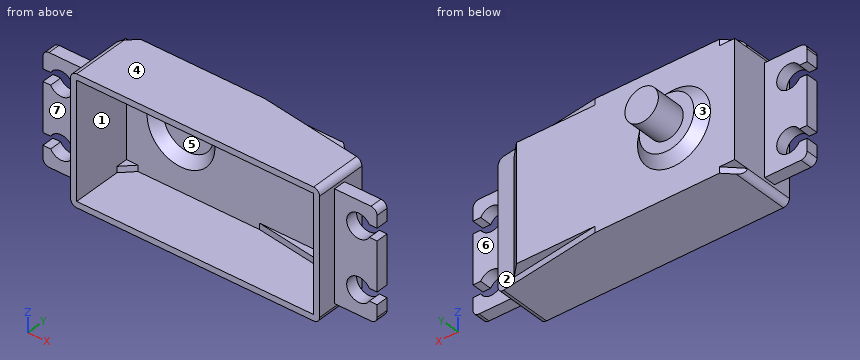
from build123d import *

# Parameters (mm, degrees)
BOSS_EXTRU_1_DEPTH      = 11
ENL_V_MAT_EXTRU_1_DEPTH = 48.360320945
ESQUISSE6_W             = 24.300768243
ESQUISSE6_H             = 19
BOSS_EXTRU_2_DEPTH      = 5
CHANFREIN1_SIZE         = 2.08
ESQUISSE7_R             = 6
BOSS_EXTRU_3_DEPTH      = 1.5
CHANFREIN2_SIZE         = 1.5
ENL_V_MAT_EXTRU_2_DEPTH = 1
ENL_V_MAT_EXTRU_3_DEPTH = 1
ESQUISSE11_W            = 18
ESQUISSE11_H            = 2
BOSS_EXTRU_4_DEPTH      = 7
ENL_V_MAT_EXTRU_5_DEPTH = 47.671725916
CONG_1_R                = 1
CONG_1_OF_SYM_TRIE1_R   = 1
COQUE1_START            = -20
COQUE1_DEPTH            = 19
COQUE1_START_2          = -19
COQUE1_2_DEPTH          = 17
ESQUISSE18_R            = 2.75
BOSS_EXTRU_5_DEPTH      = 5


with BuildPart() as part:
    # Esquisse3 → Boss.-Extru.1 (new body)
    with BuildSketch(Plane(origin=(0, 0, 0), x_dir=(1, 0, 0), z_dir=(0, 1, 0))):
        with BuildLine():
            Line((1, 0), (40, 0))
            ThreePointArc((40, 0), (40.707106781, 0.292893219), (41, 1))
            Line((41, 1), (41, 20))
            ThreePointArc((41, 20), (40.707106781, 20.707106781), (40, 21))
            Line((40, 21), (1, 21))
            ThreePointArc((1, 21), (0.292893219, 20.707106781), (0, 20))
            Line((0, 20), (0, 1))
            ThreePointArc((0, 1), (0.292893219, 0.292893219), (1, 0))
        make_face()
    extrude(amount=BOSS_EXTRU_1_DEPTH)

    # Esquisse4 → Enlèv. mat.-Extru.1 (cut, through all)
    with BuildSketch(Plane.XY):
        Polygon((41, 11), (23, 11), (41, 8.5), align=None)
    extrude(amount=-ENL_V_MAT_EXTRU_1_DEPTH, mode=Mode.SUBTRACT)

    # Esquisse6 → Boss.-Extru.2 (add)
    with BuildSketch(Plane(origin=(0, 11, 0), x_dir=(1, 0, 0), z_dir=(0, 1, 0))):
        with Locations((25.849615878, 10.5)):
            Rectangle(ESQUISSE6_W, ESQUISSE6_H)
    extrude(amount=-BOSS_EXTRU_2_DEPTH)

    # Chanfrein1
    chanfrein1_edges = [part.edges().sort_by_distance(p)[0] for p in [
        (38, 11, -10.5),
    ]]
    chamfer(chanfrein1_edges, length=CHANFREIN1_SIZE)

    # Esquisse7 → Boss.-Extru.3 (add)
    with BuildSketch(Plane(origin=(0, 11, 0), x_dir=(1, 0, 0), z_dir=(0, 1, 0))):
        with Locations(Location((10, 10.5, 0), (0, 0, 90))):
            Circle(ESQUISSE7_R)
    extrude(amount=BOSS_EXTRU_3_DEPTH)

    # Chanfrein2
    chanfrein2_edges = [part.edges().sort_by_distance(p)[0] for p in [
        (10, 12.5, -4.5),
    ]]
    chamfer(chanfrein2_edges, length=CHANFREIN2_SIZE - 0.0001)  # a hair under: the kernel refuses the full size

    # Esquisse8 → Enlèv. mat.-Extru.2 (cut)
    with BuildSketch(Plane.XY):
        Polygon((0, 11), (2.5, 11), (0, 8.5), align=None)
    extrude(amount=-ENL_V_MAT_EXTRU_2_DEPTH, mode=Mode.SUBTRACT)

    # Esquisse9 → Enlèv. mat.-Extru.3 (cut)
    with BuildSketch(Plane(origin=(0, 0, -21), x_dir=(-1, 0, 0), z_dir=(0, 0, -1))):
        Polygon((0, 11), (-2.5, 11), (0, 8.5), align=None)
    extrude(amount=-ENL_V_MAT_EXTRU_3_DEPTH, mode=Mode.SUBTRACT)

    # Esquisse11 → Boss.-Extru.4 (add)
    with BuildSketch(Plane.ZY):
        with Locations((-10.5, 4)):
            Rectangle(ESQUISSE11_W, ESQUISSE11_H)
    boss_extru_4 = extrude(amount=BOSS_EXTRU_4_DEPTH)

    # Esquisse15 → Enlèv. mat.-Extru.5 (cut, through all)
    with BuildSketch(Plane(origin=(0, 5, 0), x_dir=(1, 0, 0), z_dir=(0, 1, 0))):
        with BuildLine():
            Line((-9.636099445, 16.5), (-5.732050808, 16.5))
            ThreePointArc((-5.732050808, 16.5), (-2, 15.5), (-5.732050808, 14.5))
            Line((-5.732050808, 14.5), (-9.636099445, 14.5))
            Line((-9.636099445, 14.5), (-9.636099445, 16.5))
        make_face()
        with BuildLine():
            Line((-9.636099445, 4.5), (-5.732050808, 4.5))
            ThreePointArc((-5.732050808, 4.5), (-2, 5.5), (-5.732050808, 6.5))
            Line((-5.732050808, 6.5), (-9.636099445, 6.5))
            Line((-9.636099445, 6.5), (-9.636099445, 4.5))
        make_face()
    enl_v_mat_extru_5 = extrude(amount=-ENL_V_MAT_EXTRU_5_DEPTH, mode=Mode.SUBTRACT)

    # Congé1
    cong_1_edges = [part.edges().sort_by_distance(p)[0] for p in [
        (-7, 4, -19.5),
        (-7, 4, -1.5),
    ]]
    fillet(cong_1_edges, radius=CONG_1_R)

    # Symétrie1: Boss.-Extru.4, Enlèv. mat.-Extru.5 across plane
    add(boss_extru_4.mirror(Plane.ZY.offset(-20.5)))
    add(enl_v_mat_extru_5.mirror(Plane.ZY.offset(-20.5)), mode=Mode.SUBTRACT)

    # Congé1 of Symétrie1
    cong_1_of_sym_trie1_edges = [part.edges().sort_by_distance(p)[0] for p in [
        (48, 4, -19.5),
        (48, 4, -1.5),
    ]]
    fillet(cong_1_of_sym_trie1_edges, radius=CONG_1_OF_SYM_TRIE1_R)

    # Coque1: read off the stored shape, not the designer's step
    # Coque1 outline → Coque1 (cut)
    with BuildSketch(Plane.XY.offset(COQUE1_START)):
        Polygon((1, 8.085786438), (1, 0), (40, 0), (40, 7.629289897), (22.930887262, 10), (2.914213562, 10), align=None)
    extrude(amount=COQUE1_DEPTH, mode=Mode.SUBTRACT)

    # Coque1 2 outline → Coque1 2 (cut)
    with BuildSketch(Plane.XY.offset(COQUE1_START_2)):
        Polygon((1, 10), (1, 8.085786438), (2.914213562, 10), align=None)
        Polygon((35.505786438, 10), (22.930887262, 10), (37, 8.045956564), (37, 8.505786438), align=None)
    extrude(amount=COQUE1_2_DEPTH, mode=Mode.SUBTRACT)

    # Coque1 3 outline → Coque1 3 (revolve, cut)
    with BuildSketch(Plane(origin=(10, 0, -10.5), x_dir=(1, 0, 0), z_dir=(0, 0, 1))):
        Polygon((4.085786438, 11.5), (0, 11.5), (0, 10), (5.585786438, 10), align=None)
    revolve(axis=Axis((10, 0, -10.5), (0, 1, 0)), mode=Mode.SUBTRACT)

    # Esquisse18 → Boss.-Extru.5 (add)
    with BuildSketch(Plane(origin=(0, 12.5, 0), x_dir=(1, 0, 0), z_dir=(0, 1, 0))):
        with Locations(Location((10, 10.5, 0), (0, 0, 270))):
            Circle(ESQUISSE18_R)
    extrude(amount=BOSS_EXTRU_5_DEPTH)


solid = part.part
Source: CAD feature listing. Evaluate the final solid. Frame: model axes, mm. Face numbers are marked on the shaded views. A direction names the side the tool comes from. Give positions to 0.01 mm unless a question says otherwise; leave off trailing zeros. Write each loop counter-clockwise with the first axis right and the second up, starting at its lowest first coordinate (ties: lowest second). Pieces come first, ordered by that corner, then holes. Notation, with made-up numbers: (33.5, 64.25) -> (74.5, 64.25) arc R21 cw to (74.5, 71.25) -> close; hole circle Ø6 at (65.5, 29.5). An arc over 180 degrees is marked (long way). Return JSON: item names as keys, results as strings. Group by question number.
1. Section B-B, the plane x = 21. Output: boundary loops of the cut face in (y, z).
2. Material intervals for line 1 (Z direction, x = -4, y = 3.9); line 2 (X direction, y = 4.25, z = -5.5); line 3 (Z direction, x = 31.5, y = 2.5), sorted ascending. Write a range as from..to.
3. Section C-C, the plane y = 16.25. Output: boundary loops of the cut face in (x, z), then the cut area to 3 significant figures.
4. Access query for the marked faces 5, 6 and 7. Directions: +Z, -Z, +X, -X, +Y, -Y. A direction counts if a zero-diameter tool reaches every point of the face in a straight line with its end or side. Return the directions, or none.
5. Mould query, pull axis Z, two halves, no side actions, for the marked faces 1, 2, 3 and 4. Classes: +Z half, -Z half, draft (parallel to the pull), parting line (faces both ways), or undercut.
6. Section A-A, the plane x = -4. Output: boundary loops of the cut face in (y, z).
7. Pin query (flat end, axial travel): pin 1 Ø1.4 at (x, y) = (-6.5, 4.5) entering from +Z; pin 2 Ø0.6 at (x, y) = (-3.5, 3.5) entering from -Z; pin 3 Ø7.5 at (x, z) = (45.5, -15) entering from +Y. Return the tip coordinate at first contact, or that it passes through.
Determined:
{
 "1": {"outline": "(0, -21) -> (11, -21) -> (11, 0) -> (0, 0) -> (0, -1) -> (10, -1) -> (10, -20) -> (0, -20) -> close"},
 "2": {"line 1": "z = -19.5..-17.5, -13.5..-7.5, -3.5..-1.5", "line 2": "x = -2..1, 40..43", "line 3": "z = -21..-20, -1..0"},
 "3": {"outline": "circle Ø5.5 at (10, -10.5)", "area": "23.8 mm2"},
 "4": {"face 5": "-Y", "face 6": "+Z, -Z, +X, +Y", "face 7": "+Z, -Z, -X, -Y"},
 "5": {"face 1": "undercut", "face 2": "draft", "face 3": "parting line", "face 4": "+Z half"},
 "6": {"outline": "(3, -19.5) -> (5, -19.5) -> (5, -17.5) -> (3, -17.5) -> close; (3, -13.5) -> (5, -13.5) -> (5, -7.5) -> (3, -7.5) -> close; (3, -3.5) -> (5, -3.5) -> (5, -1.5) -> (3, -1.5) -> close"},
 "7": {"pin 1": "stops at z = -1.5", "pin 2": "stops at z = -19.5", "pin 3": "stops at y = 5"}
}
